Geometry check sheet. Reference: the model listing, model coordinates, mm. A direction names the side the tool comes from. Round coordinates to 2 decimals unless told otherwise and drop trailing zeros. Order: outer loops, then holes, each group sorted by start corner. A loop starts at its lowest first (then second) coordinate and runs counter-clockwise, first axis right, second up.
(1) Set-up check for faces 1 (the face through (-1.517, -21.972, 4.166)), 2 (the face through (29, -10, 4)): record each of +Z, -Z, +X, -X, +Y, -Y from which the full face is reachable in a straight line by a thin tool's end or side.
(2) Sectioned sample at D-D (y = -18). Record the boundary of the cut face in (x, z), plus the area to 3 significant figures.
(3) Material ranges on line 1 along Z through (x, y) = (0, -13.25); line 2 along X through (y, z) = (-14, 1.5); line 3 along X through (y, z) = (-9, 1.5), recorded low to high.
(4) Sectioned sample at A-A (y = -10). Record the boundary of the cut face in (x, z), plus the area to 3 significant figures.
(5) Release check for a two-part mould opening along X. For faces 3 (the face through (-29, -10, 4)), 4 (the face through (-0.3, -20, 3.6)), 5 (the face through (18.349, -5.043, 3.944)) record: +X half, -X half, draft (parallel to the pull), parting line (faces both ways), or undercut.
(6) Go/stop test with flat-tipped pins: pin 1 (6 mm diameter, centred on x = 0, z = 11, fed in from -Y); pin 2 (1.5 mm diameter, centred on x = -4.5, z = 3.5, fed in from -Y); pin 3 (12 mm diameter, centred on y = -17.5, z = 6, fed in from +X); pin 4 (9.5 mm diameter, centred on x = -19.5, y = -7.5, fed in from +Z). Record where each tip stops, or that it passes through.
(7) Sectioned sample at C-C (z = 11). Record the boundary of the cut face in (x, y).
(8) Sectioned sample at B-B (x = -15). Record the boundary of the cut face in (y, z).
from build123d import *

# Parameters (mm, degrees)
F0_R     = 5
F1_DEPTH = 8
F2_R     = 7
F3_DEPTH = 20
F2_R_2   = 5
F4_DEPTH = 24
F5_D     = 10
F5_DEPTH = 20
F5_TIP   = 3.0043030951


with BuildPart() as f1:
    # F0 (on Top) → F1 (new body)
    with BuildSketch(Plane.XY):
        with BuildLine():
            Line((19, 0), (0, 0))
            Line((0, 0), (-19, 0))
            ThreePointArc((-19, 0), (-29, -10), (-19, -20))
            Line((-19, -20), (0, -20))
            Line((0, -20), (19, -20))
            ThreePointArc((19, -20), (29, -10), (19, 0))
        make_face()
        with Locations((-19, -10)):
            Circle(F0_R, mode=Mode.SUBTRACT)
        with Locations((19, -10)):
            Circle(F0_R, mode=Mode.SUBTRACT)
    extrude(amount=F1_DEPTH)

    # F2 (on Front) → F3 (join)
    with BuildSketch(Plane.XZ):
        with BuildLine():
            ThreePointArc((-10, 11), (0, 1), (10, 11))
            ThreePointArc((10, 11), (0, 21), (-10, 11))
        make_face()
        with Locations((0, 11)):
            Circle(F2_R, mode=Mode.SUBTRACT)
    extrude(amount=F3_DEPTH)

    # F2 (on Front) → F4 (join)
    with BuildSketch(Plane.XZ):
        with Locations((0, 11)):
            Circle(F2_R)
        with Locations((0, 11)):
            Circle(F2_R_2, mode=Mode.SUBTRACT)
    extrude(amount=F4_DEPTH)

    # F5
    with Locations(Plane(origin=(0, 0, 0), x_dir=(1, 0, 0), z_dir=(0, 1, 0))):
        with Locations((0, -11)):
            Hole(F5_D / 2, depth=F5_DEPTH)
            with Locations((0, 0, -(F5_DEPTH + F5_TIP / 2))):  # 118° drill point
                Cone(0, F5_D / 2, F5_TIP, mode=Mode.SUBTRACT)


solid = f1.part
Answer below:
1. face 1: -Y
1. face 2: +Z, -Z, +X
2. outline: (-25, 0) - (25, 0) - (25, 8) - (9.54, 8) arc R10 ccw (long way) to (-9.54, 8) - (-25, 8) - close; hole circle Ø10 at (0, 11)
2. area: 538 mm2
3. line 1: z = 0 to 6, 16 to 21
3. line 2: x = -28.17 to -22, -16 to 16, 22 to 28.17
3. line 3: x = -28.95 to -23.9, -14.1 to 14.1, 23.9 to 28.95
4. outline: (-29, 0) - (-24, 0) - (-24, 8) - (-29, 8) - close; (-14, 0) - (14, 0) - (14, 8) - (9.54, 8) arc R10 ccw (long way) to (-9.54, 8) - (-14, 8) - close; (24, 0) - (29, 0) - (29, 8) - (24, 8) - close; hole circle Ø10 at (0, 11)
4. area: 442 mm2
5. face 3: -X half
5. face 4: draft
5. face 5: undercut
6. pin 1: passes through
6. pin 2: stops at y = -20
6. pin 3: stops at x = 28.89
6. pin 4: stops at z = 8
7. outline: (-10, -20) - (-7, -20) - (-7, -24) - (-5, -24) - (-5, 0) - (-10, 0) - close; (5, -24) - (7, -24) - (7, -20) - (10, -20) - (10, 0) - (5, 0) - close
8. outline: (-20, 0) - (-13, 0) - (-13, 8) - (-20, 8) - close; (-7, 0) - (0, 0) - (0, 8) - (-7, 8) - close
